Can you work these out from the model? Positions are in its coordinate system, mm. Face numbers are marked on the shaded views. Round coordinates to 2 decimals unless told otherwise and drop trailing zeros. Loops run counter-clockwise (first coordinate to the right, second up) from the corner with the lowest first, then second, coordinate; pieces in that order, holes last. Notation, with made-up numbers: (24.25, 13) -> (82.25, 13) arc R26 ccw to (82.25, 30) -> close; hole circle Ø8 at (59, 63.25). An arc over 180 degrees is marked (long way). Use a Markdown table: item, result.
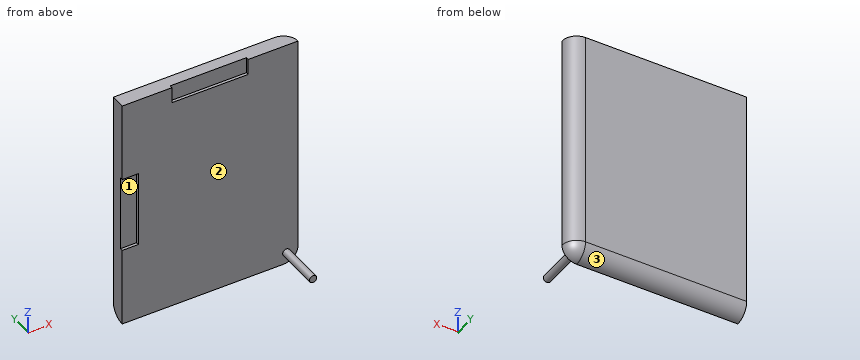
from build123d import *

# Parameters (mm, degrees)
ESQUISSE1_W             = 120
ESQUISSE1_H             = 160
BOSS_EXTRU_1_DEPTH      = 10
CONG_1_R                = 10
CONG_2_R                = 10
ESQUISSE2_R             = 2.5
BOSS_EXTRU_2_DEPTH      = 30
ESQUISSE3_W             = 11
ESQUISSE3_H             = 52
ESQUISSE3_W_2           = 52
ESQUISSE3_H_2           = 11
ENL_V_MAT_EXTRU_1_DEPTH = 2


with BuildPart() as part:
    # Esquisse1 → Boss.-Extru.1 (new body)
    with BuildSketch(Plane(origin=(0, 0, 0), x_dir=(1, 0, 0), z_dir=(0, 1, 0))):
        with Locations((60, 80)):
            Rectangle(ESQUISSE1_W, ESQUISSE1_H)
    extrude(amount=BOSS_EXTRU_1_DEPTH)

    # Congé1
    cong_1_edges = [part.edges().sort_by_distance(p)[0] for p in [
        (120, 10, -80),
    ]]
    fillet(cong_1_edges, radius=CONG_1_R - 0.0001)  # a hair under: the kernel refuses the full size

    # Congé2
    cong_2_edges = [part.edges().sort_by_distance(p)[0] for p in [
        (117.071097101, 7.071097101, -160),
        (55.00005, 10, -160),
    ]]
    fillet(cong_2_edges, radius=CONG_2_R - 0.0001)  # a hair under: the kernel refuses the full size

    # Esquisse2 → Boss.-Extru.2 (add)
    with BuildSketch(Plane.XZ):
        with Locations(Location((112, -152, 0), (0, 0, 270))):
            Circle(ESQUISSE2_R)
    extrude(amount=BOSS_EXTRU_2_DEPTH)

    # Esquisse3 → Enlèv. mat.-Extru.1 (cut)
    with BuildSketch(Plane.XZ):
        with Locations((5.5, -80)):
            Rectangle(ESQUISSE3_W, ESQUISSE3_H)
        with Locations((60, -5.5)):
            Rectangle(ESQUISSE3_W_2, ESQUISSE3_H_2)
    extrude(amount=-ENL_V_MAT_EXTRU_1_DEPTH, mode=Mode.SUBTRACT)


solid = part.part
1. If we mould it in two halves opening along Z, with no side actions, what happens to the marked faces 1, 2 and 3? For each: +Z half, -Z half, draft (parallel to the pull), parting line (faces both ways), or undercut.
Answer sheet:
| item | result |
|---|---|
| face 1 | undercut |
| face 2 | draft |
| face 3 | -Z half |
2. Will these pins go through, and if not, where does the flat tip stop? pin 1 Ø1.6 at (x, y) = (6.5, 1) entering from -Z; pin 2 Ø4 at (x, y) = (66.5, -3) entering from +Z; pin 3 Ø0.6 at (x, y) = (5, 1) entering from +Z; pin 4 Ø6 at (x, z) = (85, -78) entering from -Y.
Answer sheet:
| item | result |
|---|---|
| pin 1 | stops at z = -160 |
| pin 2 | passes through |
| pin 3 | stops at z = 0 |
| pin 4 | stops at y = 0 |
3. I need wall thicknesses on line 1 (Y direction, x = 5.5, z = -50); line 2 (Y direction, x = 51, z = -8); line 3 (Z direction, x = 68, y = 7). Which ranges of each line are inside material? Lowest first, please.
Answer sheet:
| item | result |
|---|---|
| line 1 | y = 0 to 10 |
| line 2 | y = 2 to 10 |
| line 3 | z = -157.14 to 0 |
4. I want a section at C-C (y = -23). Please give me the cut outline in (x, z).
Answer sheet:
| item | result |
|---|---|
| outline | circle Ø5 at (112, -152) |
